Solid Edge part; units mm, degrees
sketch "Sketch1" plane through (0, 0, 0) normal (0, -1, 0) x (1, 0, 0)
  circle A0 centre (0, 0) radius 12
extrude "Protrusion1" add sketch "Sketch1" against normal blind 35
sketch "Sketch2" plane through (0, 0, 0) normal (0, -1, 0) x (1, 0, 0)
  circle A0 centre (-8.5, 0) radius 1.5
  circle A1 centre (8.5, 0) radius 1.5
extrude "ExtrudedCutout_1" cut sketch "Sketch2" against normal blind 4
sketch "Sketch3" plane through (0, 0, 0) normal (0, -1, 0) x (1, 0, 0)
  circle A0 centre (0, 0) radius 1.15
extrude "ExtrudedProtrusion_2" add sketch "Sketch3" along normal blind 12
sketch "Sketch4" plane through (0, 0, 0) normal (1, 0, 0) x (0, 1, 0)
  line L0 (-12, 0.85) -> (-2, 0.85)
  line L1 (-2, 0.85) -> (-2, 1.15)
  line L2 (-12, 1.15) -> (-2, 1.15)
  line L3 (-12, 0.85) -> (-12, 1.15)
extrude "ExtrudedCutout_2" cut sketch "Sketch4" along normal mid plane 5
Design review of the part built by this model. Coordinates are the model's own, in mm. A direction names the side the tool comes from. Coordinates: 2 decimals unless noted, no trailing zeros. Loops run counter-clockwise (first coordinate to the right, second up) from the corner with the lowest first, then second, coordinate; pieces in that order, holes last.
Item 1: Clearance check with flat-ended pins moving along their axes: pin 1 (0.9 mm diameter, centred on x = -8.5, z = 0.5, fed in from -Y); pin 2 (4 mm diameter, centred on y = 11, z = 7.5, fed in from +X); pin 3 (1.5 mm diameter, centred on y = 0, z = 8.5, fed in from +X). State where each tip first meets the part, or that it passes through.
Completed:
pin 1: stops at y = 4
pin 2: stops at x = 10.67
pin 3: stops at x = 9.16
Item 2: Add section A-A (x = 0). Write out the cut boundary in (y, z).
Completed:
outline: (-12, -1.15) - (0, -1.15) - (0, -12) - (35, -12) - (35, 12) - (0, 12) - (0, 1.15) - (-2, 1.15) - (-2, 0.85) - (-12, 0.85) - close
Item 3: For faces 4 (the flat face through (0, 35, 0)), 5 (the flat face through (-8, 4, 0)), list the 3-axis set-ups (+Z, -Z, +X, -X, +Y, -Y) from which the entire face can be reached by the end or side of a thin tool; tool diameter is ignored.
Completed:
face 4: +Z, -Z, +X, -X, +Y
face 5: -Y
Item 4: Wall thickness on L1, parallel to Y at x = 0.75, z = 11; L2, parallel to Z at x = -8.5, y = 2; L3, parallel to X at y = 16.5, z = -7: over which ranges is each line inside the solid? List them lowest first.
Completed:
L1: y = 0 to 35
L2: z = -8.47 to -1.5, 1.5 to 8.47
L3: x = -9.75 to 9.75
Item 5: Draft analysis for pull direction X (two halves, no side actions). For faces 1 (the flat face through (9, 4, 0)), 2 (the cylindrical face through (-0.15, -5.92, -1.14)), 3 (the flat face through (0, -7, 0.85)), state which applies: pulls with the +X half, pulls with the -X half, needs draft (parallel to the pull), parting line crosses it, or undercut.
Completed:
face 1: undercut
face 2: parting line crosses it
face 3: needs draft
Item 6: Add section B-B (z = 0). Write out the cut boundary in (x, y), and give its area (3 significant figures).
Completed:
outline: (-12, 0) - (-10, 0) - (-10, 4) - (-7, 4) - (-7, 0) - (-1.15, 0) - (-1.15, -12) - (1.15, -12) - (1.15, 0) - (7, 0) - (7, 4) - (10, 4) - (10, 0) - (12, 0) - (12, 35) - (-12, 35) - close
area: 844 mm2
Item 7: Add section D-D (x = -8.5). Write out the cut boundary in (y, z), and give its area (3 significant figures).
Completed:
outline: (0, -8.47) - (35, -8.47) - (35, 8.47) - (0, 8.47) - (0, 1.5) - (4, 1.5) - (4, -1.5) - (0, -1.5) - close
area: 581 mm2
Item 8: Add section C-C (y = -3). Write out the cut boundary in (x, z).
Completed:
outline: (-0.77, 0.85) arc R1.15 ccw (long way) to (0.77, 0.85) - close
